from build123d import *

# Parameters (mm, degrees)
SKETCH1_R           = 52
BOSS_EXTRUDE1_DEPTH = 5
CUT_EXTRUDE3_DEPTH  = 2.4
CUT_EXTRUDE6_DEPTH  = 5
CUT_EXTRUDE7_DEPTH  = 5
CIRPATTERN1_COUNT   = 4


with BuildPart() as part:
    # Sketch1 → Boss-Extrude1 (new body)
    with BuildSketch(Plane(origin=(0, 0, 0), x_dir=(1, 0, 0), z_dir=(0, 1, 0))):
        Circle(SKETCH1_R)
    extrude(amount=BOSS_EXTRUDE1_DEPTH)

    # Sketch4 → Cut-Extrude3 (cut)
    with BuildSketch(Plane.XZ):
        Polygon((-30.27517129, 23.328400706), (-34.046075388, 26.612474905), (-32.609483493, 28.262026633), (-31.859987156, 27.61559837), (-30.422563818, 29.274773748), (-24.360613821, 24.023015245), (-26.001788353, 22.128655871), (-26.755565092, 22.781688872), (-27.999168756, 21.346233829), align=None)
        Polygon((-37.903449254, -4.912108587), (-42.892072249, -5.256349311), (-43.042657591, -3.074116227), (-42.05558984, -3.001236093), (-42.212392211, -0.811610142), (-34.212392211, -0.238718243), (-34.033363493, -2.738718243), (-35.028128199, -2.809954823), (-34.892468788, -4.704335401), align=None)
        Polygon((-4.912108587, 37.903449254), (-5.256349311, 42.892072249), (-3.074116227, 43.042657591), (-3.001236093, 42.05558984), (-0.811610142, 42.212392211), (-0.238718243, 34.212392211), (-2.738718243, 34.033363493), (-2.809954823, 35.028128199), (-4.704335401, 34.892468788), align=None)
        Polygon((23.328400706, 30.27517129), (26.612474905, 34.046075388), (28.262026633, 32.609483493), (27.61559837, 31.859987156), (29.274773748, 30.422563818), (24.023015245, 24.360613821), (22.128655871, 26.001788353), (22.781688872, 26.755565092), (21.346233829, 27.999168756), align=None)
        Polygon((37.903449254, 4.912108587), (42.892072249, 5.256349311), (43.042657591, 3.074116227), (42.05558984, 3.001236093), (42.212392211, 0.811610142), (34.212392211, 0.238718243), (34.033363493, 2.738718243), (35.028128199, 2.809954823), (34.892468788, 4.704335401), align=None)
        Polygon((30.27517129, -23.328400706), (34.046075388, -26.612474905), (32.609483493, -28.262026633), (31.859987156, -27.61559837), (30.422563818, -29.274773748), (24.360613821, -24.023015245), (26.001788353, -22.128655871), (26.755565092, -22.781688872), (27.999168756, -21.346233829), align=None)
        Polygon((4.912108587, -37.903449254), (5.256349311, -42.892072249), (3.074116227, -43.042657591), (3.001236093, -42.05558984), (0.811610142, -42.212392211), (0.238718243, -34.212392211), (2.738718243, -34.033363493), (2.809954823, -35.028128199), (4.704335401, -34.892468788), align=None)
        Polygon((-23.328400706, -30.27517129), (-26.612474905, -34.046075388), (-28.262026633, -32.609483493), (-27.61559837, -31.859987156), (-29.274773748, -30.422563818), (-24.023015245, -24.360613821), (-22.128655871, -26.001788353), (-22.781688872, -26.755565092), (-21.346233829, -27.999168756), align=None)
    extrude(amount=-CUT_EXTRUDE3_DEPTH, mode=Mode.SUBTRACT)

    # Sketch8 → Cut-Extrude6 (cut)
    with BuildSketch(Plane.XZ):
        with BuildLine():
            Line((-47.90528304, 14.320749174), (-38.443448295, 11.078076484))
            Line((-38.443448295, 11.078076484), (-37.143919852, 14.869986599))
            Line((-37.143919852, 14.869986599), (-46.600463643, 18.121721449))
            ThreePointArc((-46.600463643, 18.121721449), (-47.291076183, 16.2343498), (-47.90528304, 14.320749174))
        make_face()
        with BuildLine():
            Line((2.958916284, 14.705264854), (10.141430922, 35.593119285))
            Line((10.141430922, 35.593119285), (13.857171973, 34.31542154))
            Line((13.857171973, 34.31542154), (6.696805901, 13.422100831))
            ThreePointArc((6.696805901, 13.422100831), (4.87030494, 14.187322855), (2.958916284, 14.705264854))
        make_face()
        with BuildLine():
            Line((13.422100831, -6.696805901), (34.31542154, -13.857171973))
            Line((34.31542154, -13.857171973), (35.593119285, -10.141430922))
            Line((35.593119285, -10.141430922), (14.705264854, -2.958916284))
            ThreePointArc((14.705264854, -2.958916284), (14.187322855, -4.87030494), (13.422100831, -6.696805901))
        make_face()
        with BuildLine():
            Line((-13.893125689, -34.303058466), (-6.710611051, -13.415204036))
            ThreePointArc((-6.710611051, -13.415204036), (-4.87030494, -14.187322855), (-2.943785902, -14.708301213))
            Line((-2.943785902, -14.708301213), (-10.10547522, -35.605483041))
            Line((-10.10547522, -35.605483041), (-13.893125689, -34.303058466))
        make_face()
        with BuildLine():
            Line((-14.320749174, -47.90528304), (-11.078076484, -38.443448295))
            Line((-11.078076484, -38.443448295), (-14.869986599, -37.143919852))
            Line((-14.869986599, -37.143919852), (-18.121721449, -46.600463643))
            ThreePointArc((-18.121721449, -46.600463643), (-16.2343498, -47.291076183), (-14.320749174, -47.90528304))
        make_face()
        with BuildLine():
            Line((-35.605483041, 10.10547522), (-34.303058466, 13.893125689))
            Line((-34.303058466, 13.893125689), (-13.415204036, 6.710611051))
            ThreePointArc((-13.415204036, 6.710611051), (-14.187322855, 4.87030494), (-14.708301213, 2.943785902))
            Line((-14.708301213, 2.943785902), (-35.605483041, 10.10547522))
        make_face()
        with BuildLine():
            Line((11.116964613, 38.430120915), (14.831096483, 37.157247914))
            Line((14.831096483, 37.157247914), (18.073769174, 46.619082658))
            ThreePointArc((18.073769174, 46.619082658), (16.2343498, 47.291076183), (14.370026682, 47.890524461))
            Line((14.370026682, 47.890524461), (11.116964613, 38.430120915))
        make_face()
        with BuildLine():
            Line((38.430120915, -11.116964613), (37.157247914, -14.831096483))
            Line((37.157247914, -14.831096483), (46.619082658, -18.073769174))
            ThreePointArc((46.619082658, -18.073769174), (47.291076183, -16.2343498), (47.890524461, -14.370026682))
            Line((47.890524461, -14.370026682), (38.430120915, -11.116964613))
        make_face()
    extrude(amount=-CUT_EXTRUDE6_DEPTH, mode=Mode.SUBTRACT)

    # Sketch9 → Cut-Extrude7 (cut)
    with BuildSketch(Plane(origin=(34.948088876, 0, -12.017278305), x_dir=(0.325173485, 0, 0.945654379), z_dir=(-0.945654379, 0, 0.325173485))):
        Polygon((0.769009966, 2.5), (0.769009966, 2), (1.769009966, 2), (1.769009966, 3), (0.769009966, 3), align=None)
        Polygon((-0.730990034, 2.5), (-0.730990034, 2), (-1.730990034, 2), (-1.730990034, 3), (-0.730990034, 3), align=None)
    cut_extrude7 = extrude(amount=-CUT_EXTRUDE7_DEPTH, mode=Mode.SUBTRACT)

    # CirPattern1: Cut-Extrude7 ×4 about axis
    cirpattern1_axis = Axis((0, 0, 0), (0, 1, 0))
    for i in range(1, CIRPATTERN1_COUNT):
        add(cut_extrude7.rotate(cirpattern1_axis, i * 360 / CIRPATTERN1_COUNT), mode=Mode.SUBTRACT)


solid = part.part
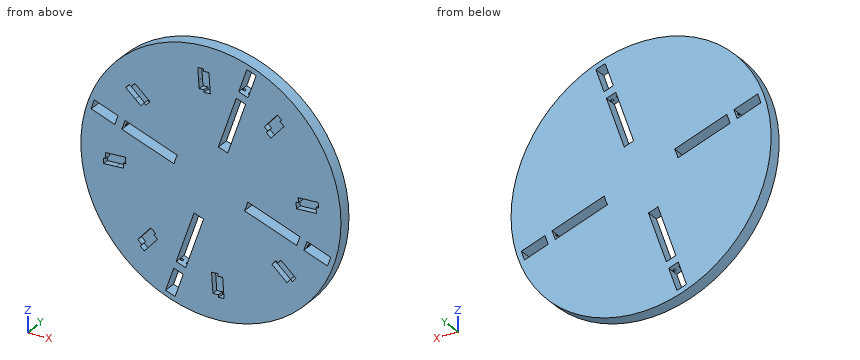
Check sheet for the modelled part. Datum: model origin and axes. Units: mm. Round coordinates to 2 decimals unless told otherwise and drop trailing zeros.
(1) Go/stop test with flat-tipped pins: P1, Ø2.5, axis at x = 40.5, z = 2, coming from the -Y side; P2, Ø1, axis at y = 1, z = -12, coming from the -X side. Record where each tip stops, or that it passes through.
(2) Cross-section at A-A, the plane y = 4. State how many separate pieces and enclosed holes the cut face has, and give its area (3 significant figures).
(3) Scan lines: probe 1 along Z at (x, y) = (-31.5, 1); probe 2 along X at (y, z) = (2.05, 22); probe 3 along Z at (x, y) = (-25.5, 1.4). Record each from-to range of solid material in increasing order.
Check sheet entries:
1. P1: stops at y = 2.4
1. P2: stops at x = -50.71
2. separate pieces: 1
2. enclosed holes: 8
2. area: 7,990 mm2
3. probe 1: z = -41.37 to 8.7, 12.93 to 24.4, 28.03 to 41.37
3. probe 2: x = -47.12 to -28.75, -27.43 to 5.47, 9.64 to 47.12
3. probe 3: z = -45.32 to -32.77, -26.07 to 6.64, 10.87 to 22.71, 25.01 to 45.32
